Source: CAD feature listing. Evaluate the final solid. Frame: model axes, mm. Face numbers are marked on the shaded views. A direction names the side the tool comes from. Give positions to 0.01 mm unless a question says otherwise; leave off trailing zeros. Loops run counter-clockwise (first coordinate to the right, second up) from the corner with the lowest first, then second, coordinate; pieces in that order, holes last.
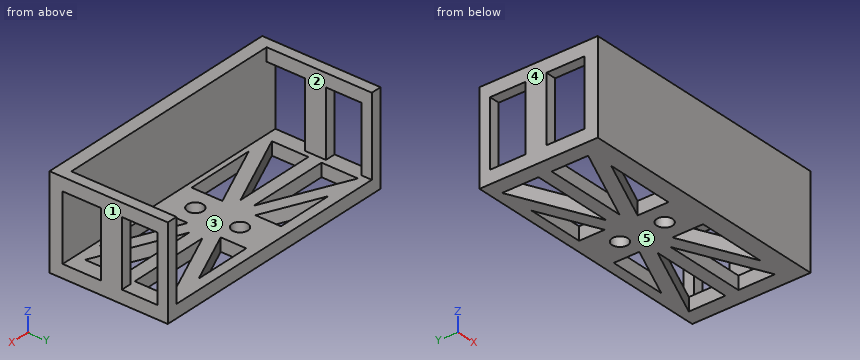
```python
from build123d import *

# Parameters (mm, degrees)
SKETCH1_W               = 90
SKETCH1_H               = 40
BOSS_EXTRUDE1_DEPTH     = 5
BOSS_EXTRUDE2_DEPTH     = 35
SKETCH3_R               = 3
CUT_EXTRUDE1_DEPTH      = 63.646443504
CUT_EXTRUDE2_DEPTH      = 35
CUT_EXTRUDE3_DEPTH      = 108.016713105
CUT_EXTRUDE3_DEPTH_BACK = 108.016713105
SKETCH5_W               = 25
SKETCH5_H               = 13.442792372
SKETCH5_H_2             = 14.528729082


with BuildPart() as part:
    # Sketch1 → Boss-Extrude1 (new body)
    with BuildSketch(Plane.XY):
        Rectangle(SKETCH1_W, SKETCH1_H)
    extrude(amount=BOSS_EXTRUDE1_DEPTH)

    # Sketch2 → Boss-Extrude2 (add)
    with BuildSketch(Plane.XY):
        Polygon((-45, 20), (-49, 20), (-49, -19.971521454), (-49, -24.971521454), (49, -24.971521454), (49, -19.971521454), (49, 20), (45, 20), (45, -19.971521454), (-45, -19.971521454), align=None)
    extrude(amount=BOSS_EXTRUDE2_DEPTH)

    # Sketch3 → Cut-Extrude1 (cut, through all)
    with BuildSketch(Plane.XY.offset(5)):
        with Locations((0, 7.028478546)):
            Circle(SKETCH3_R)
        with Locations((0, -9.971521454)):
            Circle(SKETCH3_R)
    extrude(amount=-CUT_EXTRUDE1_DEPTH, mode=Mode.SUBTRACT)

    # Sketch4 → Cut-Extrude2 (cut)
    with BuildSketch(Plane.XY.offset(5)):
        Polygon((-29.844463874, 16), (-8, 16), (-8, 6.291349389), align=None)
        Polygon((-43, 16.375317277), (-11.788929697, 2.503730476), (-43, 2.513606541), align=None)
        Polygon((-43, -2.486393709), (-11.787483748, -2.496270232), (-43, -16.348746631), align=None)
        Polygon((-8, -6.28564435), (-8, -17.971521454), (-34.330716509, -17.971521454), align=None)
        Polygon((8, -6.291349389), (8, -17.971521454), (34.280387146, -17.971521454), align=None)
        Polygon((43, -2.512973685), (43, -16.375317277), (11.788929697, -2.503730476), align=None)
        Polygon((11.787483748, 2.496270232), (43, 16.348746631), (43, 2.486393709), align=None)
        Polygon((8, 16), (29.888467798, 16), (8, 6.28564435), align=None)
    extrude(amount=-CUT_EXTRUDE2_DEPTH, mode=Mode.SUBTRACT)

    # Sketch5 → Cut-Extrude3 (cut, two sides: drawn at the far end of the back side and taken through both)
    with BuildSketch(Plane(origin=(49, 0, 0), x_dir=(0, 0, -1), z_dir=(1, 0, 0)).offset(-CUT_EXTRUDE3_DEPTH_BACK)):
        with Locations((-17.5, 9.278603814)):
            Rectangle(SKETCH5_W, SKETCH5_H)
        with Locations((-17.5, -12.707156913)):
            Rectangle(SKETCH5_W, SKETCH5_H_2)
    extrude(amount=CUT_EXTRUDE3_DEPTH + CUT_EXTRUDE3_DEPTH_BACK, mode=Mode.SUBTRACT)


solid = part.part
```
(1) Mould query, pull axis X, two halves, no side actions, for the marked faces 3, 4 and 5. Classes: pulls with the +X half, pulls with the -X half, needs draft (parallel to the pull), parting line crosses it, or undercut.
A:
face 3: undercut
face 4: pulls with the -X half
face 5: needs draft
(2) Section A-A, the plane z = 22. Return the cut outline in (x, y), then the cut area to 3 significant figures.
A:
outline: (-49, -24.97) - (49, -24.97) - (49, -19.97) - (-49, -19.97) - close; (-49, -5.44) - (-45, -5.44) - (-45, 2.56) - (-49, 2.56) - close; (-49, 16) - (-45, 16) - (-45, 20) - (-49, 20) - close; (45, -5.44) - (49, -5.44) - (49, 2.56) - (45, 2.56) - close; (45, 16) - (49, 16) - (49, 20) - (45, 20) - close
area: 586 mm2
(3) Reachability of the marked faces 1 and 2 from +Z, -Z, +X, -X, +Y, -Y: full face, straight path, thin tool, end or side. Return the list, or none.
A:
face 1: +Z, -Z, +X, +Y, -Y
face 2: +Z, +Y
(4) First-contact query: pin 1 (12 mm diameter, centred on y = -18, z = 9.5, fed in from +X); pin 2 (4 mm diameter, centred on x = -33, z = 24.5, fed in from +Y); pin 3 (2 mm diameter, centred on x = -1.5, y = 10, fed in from +Z). Flat tips, straight axial feed; report the tip coordinate or a pass-through.
A:
pin 1: stops at x = 49
pin 2: stops at y = -19.97
pin 3: stops at z = 5
(5) Section B-B, the plane x = 0. Return the cut outline in (y, z).
A:
outline: (-24.97, 0) - (-12.97, 0) - (-12.97, 5) - (-19.97, 5) - (-19.97, 35) - (-24.97, 35) - close; (-6.97, 0) - (4.03, 0) - (4.03, 5) - (-6.97, 5) - close; (10.03, 0) - (20, 0) - (20, 5) - (10.03, 5) - close
(6) Ray query, line 1 along Y through (x, z) = (0, 3); line 2 along Z through (x, y) = (11, 5.5); line 3 along X through (y, z) = (1, 32.5). Return the intervals inside material, ascending.
A:
line 1: y = -24.97 to -12.97, -6.97 to 4.03, 10.03 to 20
line 2: z = 0 to 5
line 3: x = -49 to -45, 45 to 49
(7) Section D-D, the plane y = 1. Return the cut outline in (x, z), then the cut area to 3 significant figures.
A:
outline: (-49, 0) - (49, 0) - (49, 35) - (45, 35) - (45, 5) - (-45, 5) - (-45, 35) - (-49, 35) - close
area: 730 mm2
(8) Section C-C, the plane y = -11. Count the separate pieces of the cut face and the enclosed holes in it, then the cut area to 3 significant figures.
A:
separate pieces: 8
enclosed holes: 0
area: 275 mm2
